Here's the drawing with two shaded views (mm, measured from the low corner). I have some questions. A direction names the side the tool comes from. Give positions to 0.01 mm unless a question says otherwise; leave off trailing zeros. Order: outer loops, then holes, each group sorted by start corner. A loop starts at its lowest first (then second) coordinate and runs counter-clockwise, first axis right, second up. Notation, with made-up numbers: (-39.5, 10) - (10.5, 10) arc R21 ccw to (10.5, 18) - close; hole circle Ø7 at (15.25, 32). An arc over 180 degrees is marked (long way). Use one line per item in the form item = value. Start each with the question number.
1) Suppose I cut it at A-A, the plane z = 43.65. State how many separate pieces and enclosed holes the cut face has, and give its area (3 significant figures).
2) We'd pull the mould along Y, two halves only. Please class the marked faces 1, 2 and 3: released by +Y, released by -Y, zero draft, split by the parting line, or undercut.
3) For pin 1 (1.5 mm diameter, centred on x = 12.5, z = 12, fed in from -Y); pin 2 (3 mm diameter, centred on x = 5, z = 43.65, fed in from +Y); pin 3 (3.5 mm diameter, centred on x = 13.5, y = 17, fed in from +Z); pin 4 (4 mm diameter, centred on x = 16, z = 43.65, fed in from -Y) (3 decimals), each with a flat end and sliding along its axis, tell me the tip position at first contact or that it passes through.
4) Suppose I cut it at C-C, the plane z = 10. Write out the boundary of the cut face in (x, y).
5) Please list where these lines run through material, in increasing order: probe 1 along Y at (x, z) = (12.5, 6); probe 2 along X at (y, z) = (28, 43); probe 3 along X at (y, z) = (9, 43).
6) Which directions (+Z, -Z, +X, -X, +Y, -Y) give clear straight access to the entire face, cutting with the end or side of a thin tool? Please do the marked faces 4 and 5.
7) Suppose I cut it at B-B, the plane x = 5. Write out the boundary of the cut face in (y, z) (3 decimals).
8) Suppose I cut it at D-D, the plane y = 30.5. Write out the boundary of the cut face in (x, z), and give its area (3 significant figures).
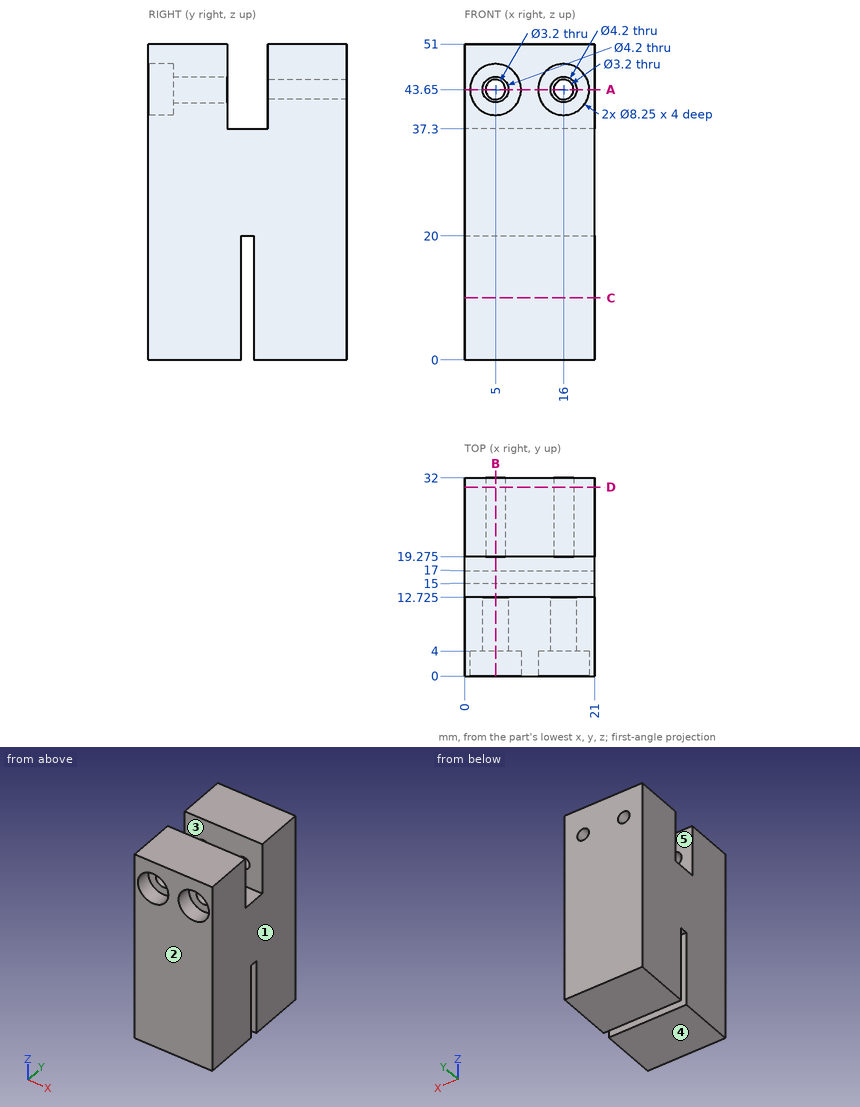
Result sheet:
q1.separate_pieces = 6
q1.enclosed_holes = 0
q1.area = 314 mm²
q2.face_1 = zero draft
q2.face_2 = released by -Y
q2.face_3 = undercut
q3.pin_1 = 0
q3.pin_2 = through
q3.pin_3 = 37.3
q3.pin_4 = 19.275
q4.outline = (0, 0) - (21, 0) - (21, 15) - (0, 15) - close; (0, 17) - (21, 17) - (21, 32) - (0, 32) - close
q5.probe_1 = 0 to 15, 17 to 32
q5.probe_2 = 0 to 3.54, 6.46 to 14.54, 17.46 to 21
q5.probe_3 = 0 to 3, 7 to 14, 18 to 21
q6.face_4 = -Z, +X, -X, +Y, -Y
q6.face_5 = +Z, +X, -X
q7.outline = (0, 0) - (15, 0) - (15, 20) - (17, 20) - (17, 0) - (32, 0) - (32, 42.05) - (19.275, 42.05) - (19.275, 37.3) - (12.725, 37.3) - (12.725, 41.55) - (4, 41.55) - (4, 39.525) - (0, 39.525) - close; (0, 47.775) - (4, 47.775) - (4, 45.75) - (12.725, 45.75) - (12.725, 51) - (0, 51) - close; (19.275, 45.25) - (32, 45.25) - (32, 51) - (19.275, 51) - close
q8.outline = (0, 0) - (21, 0) - (21, 51) - (0, 51) - close; hole circle Ø3.2 at (5, 43.65); hole circle Ø3.2 at (16, 43.65)
q8.area = 1,050 mm²
